Geometry: final body of the model. Coordinates: model frame, mm. Face numbers are marked on the shaded views. A direction names the side the tool comes from. Give positions to 0.01 mm unless a question says otherwise; leave off trailing zeros. Order: outer loops, then holes, each group sorted by start corner. A loop starts at its lowest first (then second) coordinate and runs counter-clockwise, first axis right, second up. Notation, with made-up numbers: (-25, 60.5) -> (17, 60.5) arc R11 cw to (17, 68.5) -> close; hole circle Ø3 at (70.25, 24). An arc over 180 degrees is marked (long way). Answer in a Markdown table with one row per item. Add a question column.
Q1. Set-up query: the marked faces 4, 5 and 6. Return all of +Z, -Z, +X, -X, +Y, -Y with unobstructed straight access to the full face (end or side cutting, diameter ignored); none if empty.
Q2. Pull-direction query (Z, two-part tool) for the marked faces 1, 2 and 3; classes: +Z half, -Z half, draft (parallel to the pull), parting line (faces both ways), or undercut.
Q3. Line query: line 1 along X through (y, z) = (3.85, -7.5); line 2 along Y through (x, z) = (-7.25, 2); line 3 along Z through (x, y) = (-2, 0.2). Output: solid intervals per line, ascending. Write a range as from..to.
Q4. Cut plane C-C on y = 1.8. Return the cut outline in (x, z), and give its area (3 significant figures).
Q5. Cut plane A-A on z = -1. Return the cut outline in (x, y).
Q6. Contact query for a flat-ended pin moving along its axis: P1, Ø1.5, axis at y = 2, z = -0.5, coming from the -X side. Output: stop coordinate, or through.
Q7. Cut plane B-B on x = 0. Return the cut outline in (y, z), and give its area (3 significant figures).
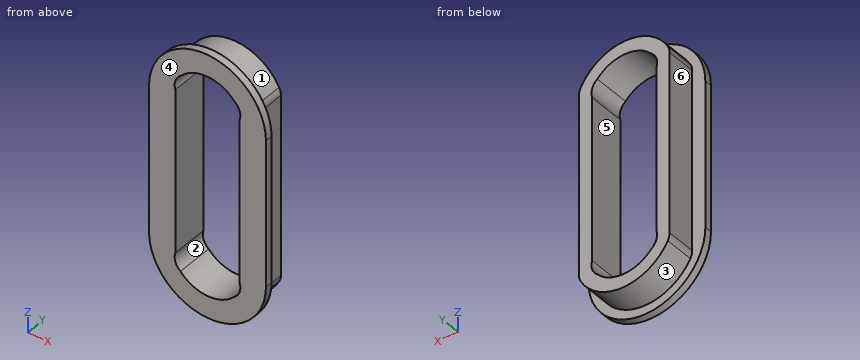
Autodesk Inventor part; units mm, degrees
ref_plane "YZ Plane" through (0, 0, 0) normal (1, 0, 0) x (0, 1, 0)
ref_plane "XZ Plane" through (0, 0, 0) normal (0, 1, 0) x (-1, 0, 0)
ref_plane "XY Plane" through (0, 0, 0) normal (0, 0, 1) x (1, 0, 0)
sketch "Sketch1" plane through (0, 0, 0) normal (0, 1, 0) x (-1, 0, 0)
  line L0 (6.25, 12.8036) -> (6.25, -12.8036) construction
  arc A0 (6.25, 12.8036) -> (-6.25, 12.8036) centre (0, 10) ccw construction
  arc A1 (4.4, 12.3749) -> (-4.4, 12.3749) centre (0, 10) ccw
  line L1 (4.4, 12.3749) -> (4.4, -12.3749)
  line L2 (-6.25, 12.8036) -> (-6.25, -12.8036) construction
  arc A2 (-6.25, -12.8036) -> (6.25, -12.8036) centre (0, -10) ccw construction
  arc A3 (-4.4, -12.3749) -> (4.4, -12.3749) centre (0, -10) ccw
  line L3 (-8, 0) -> (8, 0) construction
  circle A4 centre (0, -10) radius 7 construction
  arc A5 (3.6981, -13.3651) -> (4.4, -11.1611) centre (2.4943, -11.768) ccw
  line L4 (-4.4, 12.3749) -> (-4.4, -12.3749)
  arc A6 (-4.4, -11.1611) -> (-3.6981, -13.3651) centre (-2.4943, -11.768) ccw
  arc A7 (4.4, 11.1611) -> (3.6981, 13.3651) centre (2.4943, 11.768) ccw
  arc A8 (-3.6981, 13.3651) -> (-4.4, 11.1611) centre (-2.4943, 11.768) ccw
  arc A9 (-8, -10) -> (8, -10) centre (0, -10) ccw
  line L5 (8, -10) -> (8, 10)
  arc A10 (8, 10) -> (-8, 10) centre (0, 10) ccw
  line L6 (0, 10) -> (0, -10)
  line L7 (6.2, -12.7928) -> (6.2, 12.7928)
  arc A11 (6.2, 12.7928) -> (-6.2, 12.7928) centre (0, 10) ccw
  line L8 (-6.2, -12.7928) -> (-6.2, 12.7928)
  arc A12 (-6.2, -12.7928) -> (6.2, -12.7928) centre (0, -10) ccw
  line L9 (-8, -10) -> (-8, 10)
  point P0 (0, 0)
  point P1 (0, 0)
  point P2 (-3.6981, -13.3651)
  point P3 (4.4, 11.1611)
  point P4 (-6.2, -12.7928)
  dimension "d5" = 12.5
  dimension "d0" = 14
  dimension "d1" = 2
  dimension "d2" = 1
  dimension "d3" = 20
  dimension "d4" = 8.8
  dimension "d7" = 1.85
  dimension "d8" = 5
  dimension "d14" = 0.05
  dimension "d15" = 0.05
extrude "Extrusion1" add sketch "Sketch1" along normal blind 5 contours A12 L8 A11 L7
extrude "Extrusion2" add sketch "Sketch1" along normal blind 1 contours L9 A10 L5 A9
fillet "Fillet1" radius 2 4 edges at (6.2, 3, 12.7928) (6.2, 3, -12.7928) (-6.2, 3, -12.7928) (-6.2, 3, 12.7928)
equation "\"d7\" = -0.5 * d4 + 0.5 * d5"
equation "\"d15\" = d14"
properties part number "SliderProtectionFrame" material "Aluminum 7075"
Completed:
| question | item | result |
|---|---|---|
| 1 | face 4 | +Z, -Z, +X, -X, -Y |
| 1 | face 5 | +Y, -Y |
| 1 | face 6 | +Z, -Z, -X, +Y |
| 2 | face 1 | +Z half |
| 2 | face 2 | undercut |
| 2 | face 3 | -Z half |
| 3 | line 1 | x = -6.2..-4.4, 4.4..6.2 |
| 3 | line 2 | y = 0..1 |
| 3 | line 3 | z = -17.75..-14.58, 14.58..17.75 |
| 4 | outline | (-6.2, -12.32) arc R2 ccw to (-5.95, -13.29) arc R6.8 ccw to (5.95, -13.29) arc R2 ccw to (6.2, -12.32) -> (6.2, 12.32) arc R2 ccw to (5.95, 13.29) arc R6.8 ccw to (-5.95, 13.29) arc R2 ccw to (-6.2, 12.32) -> close; hole (-4.4, -11.16) arc R2 ccw to (-3.7, -13.37) arc R5 ccw to (3.7, -13.37) arc R2 ccw to (4.4, -11.16) -> (4.4, 11.16) arc R2 ccw to (3.7, 13.37) arc R5 ccw to (-3.7, 13.37) arc R2 ccw to (-4.4, 11.16) -> close |
| 4 | area | 137 mm² |
| 5 | outline | (-8, 0) -> (-4.4, 0) -> (-4.4, 5) -> (-6.2, 5) -> (-6.2, 1) -> (-8, 1) -> close; (4.4, 0) -> (8, 0) -> (8, 1) -> (6.2, 1) -> (6.2, 5) -> (4.4, 5) -> close |
| 6 | P1 | stops at x = -6.2 |
| 7 | outline | (0, -18) -> (1, -18) -> (1, -16.8) -> (5, -16.8) -> (5, -15) -> (0, -15) -> close; (0, 15) -> (5, 15) -> (5, 16.8) -> (1, 16.8) -> (1, 18) -> (0, 18) -> close |
| 7 | area | 20.4 mm² |
